Build history of the part. All positions in model axes, mm. A direction names the side the tool comes from. Round coordinates to 2 decimals unless told otherwise and drop trailing zeros. Loops run counter-clockwise (first coordinate to the right, second up) from the corner with the lowest first, then second, coordinate; pieces in that order, holes last. Notation, with made-up numbers: (86.5, 54) - (100.5, 54) arc R8 cw to (100.5, 60) - close; hole circle Ø5 at (12, 44.25). An arc over 180 degrees is marked (long way). Use a Markdown table: item, result.
from build123d import *

# Parameters (mm, degrees)
SKETCH1_R           = 22.479
BOSS_EXTRUDE1_DEPTH = 19.05
TWOHOLE_REACH       = 98.838
SKETCH4_R           = 3.3655


with BuildPart() as part:
    # Sketch1 → Boss-Extrude1 (new, symmetric)
    with BuildSketch(Plane(origin=(0, 0, 0), x_dir=(0, 0, -1), z_dir=(1, 0, 0))):
        with BuildLine():
            Line((0, 28.321), (76.2, 28.321))
            Line((76.2, 28.321), (76.2, 27.686))
            Line((76.2, 27.686), (5.963593296, 27.686))
            ThreePointArc((5.963593296, 27.686), (-2.998652614, -28.161802561), (0, 28.321))
        make_face()
        with Locations(Location((0, 0, 0), (0, 0, 180))):
            Circle(SKETCH1_R, mode=Mode.SUBTRACT)
    extrude(amount=BOSS_EXTRUDE1_DEPTH, both=True)

    # Sketch4 → TwoHole (cut, up to next)
    with BuildSketch(Plane(origin=(0, 28.321, 0), x_dir=(1, 0, 0), z_dir=(0, 1, 0)), mode=Mode.PRIVATE) as twohole_sk1:
        with Locations(Location((-9.525, 60.325, 0), (0, 0, 270))):
            Circle(SKETCH4_R)
    twohole_tool1 = extrude(twohole_sk1.sketch, amount=-TWOHOLE_REACH, mode=Mode.PRIVATE) & part.part
    # Sketch4 → TwoHole (cut, up to next)
    with BuildSketch(Plane(origin=(0, 28.321, 0), x_dir=(1, 0, 0), z_dir=(0, 1, 0)), mode=Mode.PRIVATE) as twohole_sk2:
        with Locations(Location((9.525, 60.325, 0), (0, 0, 270))):
            Circle(SKETCH4_R)
    twohole_tool2 = extrude(twohole_sk2.sketch, amount=-TWOHOLE_REACH, mode=Mode.PRIVATE) & part.part
    add(twohole_tool1.solids().sort_by_distance((-9.525, 28.321, -60.325))[0], mode=Mode.SUBTRACT)
    add(twohole_tool2.solids().sort_by_distance((9.525, 28.321, -60.325))[0], mode=Mode.SUBTRACT)


solid = part.part
Q1. Cut at B-B, the plane x = -3.5. List the corners of the cut face in (y, z), plus the area to 3 significant figures.
Results found:
| item | result |
|---|---|
| outline | (27.69, -76.2) - (28.32, -76.2) - (28.32, 0) arc R28.32 ccw (long way) to (27.69, -5.96) - close; hole circle Ø44.96 at (0, 0) |
| area | 978 mm2 |
Q2. Drop flat-ended pins along their axis: pin 1 (4 mm diameter, centred on x = -8, z = -54, fed in from -Y); pin 2 (1 mm diameter, centred on x = 7, y = 12.5, fed in from -Z); pin 3 (3 mm diameter, centred on x = 9, y = -21, fed in from -Z); pin 4 (8 mm diameter, centred on y = -19.5, z = 2, fed in from +X). Give the stop position or say it passes through.
Results found:
| item | result |
|---|---|
| pin 1 | stops at y = 27.69 |
| pin 2 | stops at z = -25.65 |
| pin 3 | stops at z = -20.54 |
| pin 4 | stops at x = 19.05 |
Q3. Cut at C-C, the plane z = -10.5. List the corners of the cut face in (x, y), plus the area to 3 significant figures.
Results found:
| item | result |
|---|---|
| outline | (-19.05, -26.3) - (19.05, -26.3) - (19.05, -19.88) - (-19.05, -19.88) - close; (-19.05, 19.88) - (19.05, 19.88) - (19.05, 26.3) - (-19.05, 26.3) - close; (-19.05, 27.69) - (19.05, 27.69) - (19.05, 28.32) - (-19.05, 28.32) - close |
| area | 514 mm2 |
Q4. Cut at D-D, the plane y = -17.5. List the corners of the cut face in (x, z), plus the area to 3 significant figures.
Results found:
| item | result |
|---|---|
| outline | (-19.05, -22.27) - (19.05, -22.27) - (19.05, -14.11) - (-19.05, -14.11) - close; (-19.05, 14.11) - (19.05, 14.11) - (19.05, 22.27) - (-19.05, 22.27) - close |
| area | 622 mm2 |
Q5. Cut at A-A, the plane y = 0. List the corners of the cut face in (x, z), plus the area to 3 significant figures.
Results found:
| item | result |
|---|---|
| outline | (-19.05, -28.32) - (19.05, -28.32) - (19.05, -22.48) - (-19.05, -22.48) - close; (-19.05, 22.48) - (19.05, 22.48) - (19.05, 28.32) - (-19.05, 28.32) - close |
| area | 445 mm2 |
Q6. Which spindle directions (+Z, -Z, +X, -X, +Y, -Y) get a long thin tool onto all of the face, cutting with end or side? Do faces 1 (the face through (6.24, 28.01, -61.05)), 2 (the face through (0, 27.686, -42)). Say none if no direction does.
Results found:
| item | result |
|---|---|
| face 1 | +Y, -Y |
| face 2 | -Z, +X, -X |
Q7. Probe line 1 (Z direction, x = 8, y = 1); line 2 (Y direction, x = 7.5, z = -20); line 3 (Z direction, x = -14, y = -8.5). List the from-to ranges inside material, lowest first.
Results found:
| item | result |
|---|---|
| line 1 | z = -28.3 to -22.46, 22.46 to 28.3 |
| line 2 | y = -20.05 to -10.26, 10.26 to 20.05, 27.69 to 28.32 |
| line 3 | z = -27.02 to -20.81, 20.81 to 27.02 |
Q8. Pull direction Y, two halves, no side cores. Call faces 3 (the face through (0, 28.321, -38)), 4 (the face through (0.267, -28.264, 1.8)), 5 (the face through (-0.267, 21.944, -4.873)), 6 (the face through (19.05, 21, -9)): pulls with the +Y half, pulls with the -Y half, needs draft (parallel to the pull), parting line crosses it, or undercut.
Results found:
| item | result |
|---|---|
| face 3 | pulls with the +Y half |
| face 4 | undercut |
| face 5 | undercut |
| face 6 | needs draft |
